```python
from build123d import *

# Parameters (mm, degrees)
F0_R     = 2.5
F1_DEPTH = 0.75


with BuildPart() as f1:
    # F0 (on Top) → F1 (new body, symmetric)
    with BuildSketch(Plane.XY):
        with BuildLine():
            Line((-10, 7.5), (-41, 7.5))
            Line((-41, 7.5), (-41, -7.5))
            Line((-41, -7.5), (41, -7.5))
            Line((41, -7.5), (41, 7.5))
            Line((41, 7.5), (10, 7.5))
            Line((10, 7.5), (10, 15))
            ThreePointArc((10, 15), (0, 25), (-10, 15))
            Line((-10, 15), (-10, 7.5))
        make_face()
        with Locations((-31, 0)):
            Circle(F0_R, mode=Mode.SUBTRACT)
        Circle(F0_R, mode=Mode.SUBTRACT)
        with Locations((31, 0)):
            Circle(F0_R, mode=Mode.SUBTRACT)
        with Locations((0, 15)):
            Circle(F0_R, mode=Mode.SUBTRACT)
    extrude(amount=F1_DEPTH, both=True)


solid = f1.part
```
The model under review builds one solid part; all positions refer to its coordinate system, in mm. A direction names the side the tool comes from. Round coordinates to 2 decimals unless told otherwise and drop trailing zeros. Loops run counter-clockwise (first coordinate to the right, second up) from the corner with the lowest first, then second, coordinate; pieces in that order, holes last. Notation, with made-up numbers: (86.5, 33.25) -> (107.5, 33.25) arc R20 ccw to (107.5, 65.25) -> close; hole circle Ø3 at (-4, 87). An arc over 180 degrees is marked (long way). Answer in a Markdown table with one row per item.
1) Consider section A-A, the plane x = 31. Write out the cut boundary in (y, z), plus the area to 3 significant figures.
Taken from the geometry:
| item | result |
|---|---|
| outline | (-7.5, -0.75) -> (-2.5, -0.75) -> (-2.5, 0.75) -> (-7.5, 0.75) -> close; (2.5, -0.75) -> (7.5, -0.75) -> (7.5, 0.75) -> (2.5, 0.75) -> close |
| area | 15.0 mm² |
2) Draft analysis for pull direction X (two halves, no side actions). For faces 4 (the cylindrical face through (-0.54, -2.44, -0.01)), 5 (the flat face through (-25, 7.5, 0)), 6 (the flat face through (10, 11, 0)), state which applies: pulls with the +X half, pulls with the -X half, needs draft (parallel to the pull), parting line crosses it, or undercut.
Taken from the geometry:
| item | result |
|---|---|
| face 4 | undercut |
| face 5 | needs draft |
| face 6 | pulls with the +X half |
3) Consider section B-B, the plane y = 0. Write out the cut boundary in (x, z), plus the area to 4 significant figures.
Taken from the geometry:
| item | result |
|---|---|
| outline | (-41, -0.75) -> (-33.5, -0.75) -> (-33.5, 0.75) -> (-41, 0.75) -> close; (-28.5, -0.75) -> (-2.5, -0.75) -> (-2.5, 0.75) -> (-28.5, 0.75) -> close; (2.5, -0.75) -> (28.5, -0.75) -> (28.5, 0.75) -> (2.5, 0.75) -> close; (33.5, -0.75) -> (41, -0.75) -> (41, 0.75) -> (33.5, 0.75) -> close |
| area | 100.5 mm² |
4) Tool access review of faces 1 (the flat face through (-1, 5, -0.75)), 2 (the flat face through (26, 7.5, 0)), 3 (the flat face through (-10, 11, 0)): name each direction out of +Z, -Z, +X, -X, +Y, -Y from which nothing blocks a thin tool from reaching the whole face with its end or side.
Taken from the geometry:
| item | result |
|---|---|
| face 1 | -Z, +X, -X, +Y, -Y |
| face 2 | +Z, -Z, +X, +Y |
| face 3 | +Z, -Z, -X, +Y |
5) Wall thickness on line 1 along Y through (x, z) = (0, 0); line 2 along X through (y, z) = (1, -0.45); line 3 along Y through (x, z) = (31, 0.15): over which ranges is each line inside the solid? List them lowest first.
Taken from the geometry:
| item | result |
|---|---|
| line 1 | y = -7.5 to -2.5, 2.5 to 12.5, 17.5 to 25 |
| line 2 | x = -41 to -33.29, -28.71 to -2.29, 2.29 to 28.71, 33.29 to 41 |
| line 3 | y = -7.5 to -2.5, 2.5 to 7.5 |
6) Consider section C-C, the plane z = -0.05. Write out the cut boundary in (x, y).
Taken from the geometry:
| item | result |
|---|---|
| outline | (-41, -7.5) -> (41, -7.5) -> (41, 7.5) -> (10, 7.5) -> (10, 15) arc R10 ccw to (-10, 15) -> (-10, 7.5) -> (-41, 7.5) -> close; hole circle Ø5 at (-31, 0); hole circle Ø5 at (0, 0); hole circle Ø5 at (0, 15); hole circle Ø5 at (31, 0) |
7) Consider section D-D, the plane x = 0. Write out the cut boundary in (y, z), plus the area to 4 significant figures.
Taken from the geometry:
| item | result |
|---|---|
| outline | (-7.5, -0.75) -> (-2.5, -0.75) -> (-2.5, 0.75) -> (-7.5, 0.75) -> close; (2.5, -0.75) -> (12.5, -0.75) -> (12.5, 0.75) -> (2.5, 0.75) -> close; (17.5, -0.75) -> (25, -0.75) -> (25, 0.75) -> (17.5, 0.75) -> close |
| area | 33.75 mm² |
